Input: part model. Units: mm. Frame: model coordinates. A direction names the side the tool comes from. Round coordinates to 2 decimals unless told otherwise and drop trailing zeros. Write each loop counter-clockwise with the first axis right and the second up, starting at its lowest first coordinate (ties: lowest second). Pieces come first, ordered by that corner, then holes. Notation, with made-up numbers: (9, 25) - (17, 25) arc R18 cw to (17, 38) - close; hole circle Ø5 at (-6, 31.25). An arc over 180 degrees is marked (long way). One line per item, written item: value. Start each with the question number.
```python
from build123d import *

# Parameters (mm, degrees)
SKETCH1_R           = 53.5
BOSS_EXTRUDE1_DEPTH = 2
SKETCH2_R           = 53.5
SKETCH2_R_2         = 51.6
BOSS_EXTRUDE2_DEPTH = 10
BOSS_EXTRUDE3_START = 9
SKETCH4_R           = 53.5
BOSS_EXTRUDE3_DEPTH = 9
SKETCH6_W           = 36
SKETCH6_H           = 36
CUT_EXTRUDE1_DEPTH  = 6.5
DRAFT4_START        = -19
DRAFT4_DEPTH        = 37
DRAFT4_2_DEPTH      = 38
CUT_EXTRUDE2_DEPTH  = 40.5
SKETCH14_R          = 2.35
CUT_EXTRUDE3_DEPTH  = 4


with BuildPart() as part:
    # Sketch1 → Boss-Extrude1 (new body)
    with BuildSketch(Plane(origin=(0, 0, 0), x_dir=(1, 0, 0), z_dir=(0, 1, 0))):
        with Locations(Location((0, 0, 0), (0, 0, 270))):
            Circle(SKETCH1_R)
    extrude(amount=BOSS_EXTRUDE1_DEPTH)

    # Sketch2 → Boss-Extrude2 (add)
    with BuildSketch(Plane(origin=(0, 2, 0), x_dir=(1, 0, 0), z_dir=(0, 1, 0))):
        with Locations(Location((0, 0, 0), (0, 0, 270))):
            Circle(SKETCH2_R)
        with Locations(Location((0, 0, 0), (0, 0, 270))):
            Circle(SKETCH2_R_2, mode=Mode.SUBTRACT)
    extrude(amount=BOSS_EXTRUDE2_DEPTH)

    # Sketch4 → Boss-Extrude3 (add)
    with BuildSketch(Plane.XZ.offset(BOSS_EXTRUDE3_START)):
        with Locations(Location((0, 0, 0), (0, 0, 270))):
            Circle(SKETCH4_R)
    extrude(amount=-BOSS_EXTRUDE3_DEPTH)

    # Sketch6 → Cut-Extrude1 (cut)
    with BuildSketch(Plane.XZ.offset(9)):
        Rectangle(SKETCH6_W, SKETCH6_H)
    extrude(amount=-CUT_EXTRUDE1_DEPTH, mode=Mode.SUBTRACT)

    # Draft4: read off the stored shape, not the designer's step
    # Draft4 outline → Draft4 (add)
    with BuildSketch(Plane.XY.offset(DRAFT4_START)):
        Polygon((18, -9), (18, -2.5), (15.634193477, -9), align=None)
        Polygon((-18, -9), (-15.634193477, -9), (-18, -2.5), align=None)
    extrude(amount=DRAFT4_DEPTH)

    # Draft4 2 outline → Draft4 2 (add)
    with BuildSketch(Plane.YZ.offset(DRAFT4_START)):
        Polygon((-9, 18), (-9, 15.634193477), (-2.5, 18), align=None)
    extrude(amount=DRAFT4_2_DEPTH)

    # Sketch13 → Cut-Extrude2 (cut)
    with BuildSketch(Plane.XY.offset(-18)):
        Polygon((15.634193477, -9), (-15.634193477, -9), (-18, -2.5), (18, -2.5), align=None)
    extrude(amount=-CUT_EXTRUDE2_DEPTH, mode=Mode.SUBTRACT)

    # Sketch14 → Cut-Extrude3 (cut)
    with BuildSketch(Plane.XZ.offset(2.5)):
        with Locations(Location((0, -37, 0), (0, 0, 270))):
            Circle(SKETCH14_R)
    extrude(amount=-CUT_EXTRUDE3_DEPTH, mode=Mode.SUBTRACT)


solid = part.part
```
Q1. Contact query for flat-ended pins moving along their axis: pin 1 Ø3 at (x, y) = (-42, 5) entering from -Z; pin 2 Ø11 at (x, z) = (-5.5, -32.5) entering from -Y; pin 3 Ø12 at (x, y) = (-30.5, 0) entering from +Z. Output: stop coordinate, or through.
Q2. Pull-direction query (X, two-part tool) for faces 4 (the cylindrical face through (53.384, -0.98, -3.527)), 5 (the flat face through (1, -9, 25)), 6 (the cylindrical face through (-50.373, 6.93, -11.186)); classes: pulls with the +X half, pulls with the -X half, needs draft (parallel to the pull), parting line crosses it, or undercut.
Q3. Cut plane B-B, the plane z = 0. Output: boundary loops of the cut face in (x, y), and give its area (3 significant figures).
Q4. Cut plane C-C, the plane y = 10.5. Output: boundary loops of the cut face in (x, z).
Q5. Access query for faces 1 (the flat face through (1, 2, -1)), 2 (the flat face through (-16.8, -5.8, -17.1)), 3 (the flat face through (0, 1.5, -37)). Directions: +Z, -Z, +X, -X, +Y, -Y. A direction counts if a zero-diameter tool reaches every point of the face in a straight line with its end or side. Return the directions, or none.
Q6. Cut plane A-A, the plane x = 0. Output: boundary loops of the cut face in (y, z).
Q7. Cut plane D-D, the plane z = 43. Output: boundary loops of the cut face in (x, y).
Q8. Material intervals for probe 1 along X at (y, z) = (5.25, 0); probe 2 along Y at (x, z) = (45.5, -13.5); probe 3 along X at (y, z) = (4, -31), sorted ascending. Write a range as from..to.
A:
1. pin 1: stops at z = -34.96
1. pin 2: stops at y = -2.5
1. pin 3: stops at z = 47.56
2. face 4: parting line crosses it
2. face 5: needs draft
2. face 6: undercut
3. outline: (-53.5, -9) - (-15.63, -9) - (-18, -2.5) - (18, -2.5) - (15.63, -9) - (53.5, -9) - (53.5, 12) - (51.6, 12) - (51.6, 2) - (-51.6, 2) - (-51.6, 12) - (-53.5, 12) - close
3. area: 996 mm²
4. outline: circle Ø107 at (0, 0); hole circle Ø103.2 at (0, 0)
5. face 1: +Y
5. face 2: -Z
5. face 3: -Y
6. outline: (-9, 15.63) - (-2.5, 18) - (-2.5, -34.65) - (1.5, -34.65) - (1.5, -39.35) - (-2.5, -39.35) - (-2.5, -53.5) - (12, -53.5) - (12, -51.6) - (2, -51.6) - (2, 51.6) - (12, 51.6) - (12, 53.5) - (-9, 53.5) - close
7. outline: (-31.83, -9) - (31.83, -9) - (31.83, 12) - (28.52, 12) - (28.52, 2) - (-28.52, 2) - (-28.52, 12) - (-31.83, 12) - close
8. probe 1: x = -53.5..-51.6, 51.6..53.5
8. probe 2: y = -9..2
8. probe 3: x = -43.6..-41.25, 41.25..43.6
